Input: part model. Units: mm. Frame: model coordinates. Give positions to 0.01 mm unless a question says otherwise; leave off trailing zeros. Loops run counter-clockwise (first coordinate to the right, second up) from the corner with the lowest first, then second, coordinate; pieces in that order, holes last. Notation, with made-up numbers: (39, 73.25) - (85, 73.25) arc R21 cw to (85, 98.25) - close; hole circle Ø10 at (0.5, -25.5). An arc over 180 degrees is marked (long way). One line per item, written item: value.
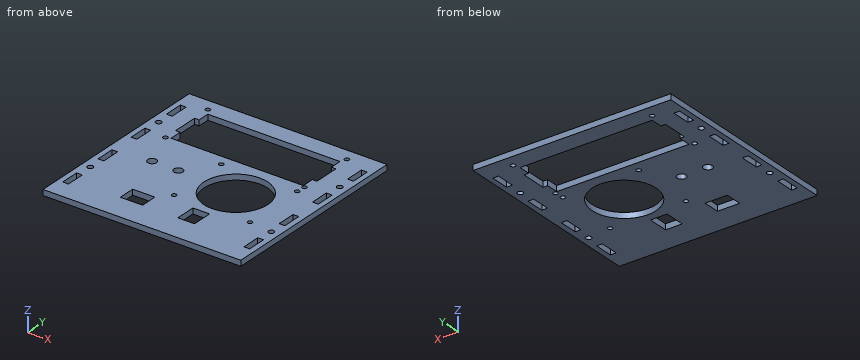
Autodesk Inventor part; units mm, degrees
ref_plane "YZ Plane" through (0, 0, 0) normal (1, 0, 0) x (0, 1, 0)
ref_plane "XZ Plane" through (0, 0, 0) normal (0, 1, 0) x (-1, 0, 0)
ref_plane "XY Plane" through (0, 0, 0) normal (0, 0, 1) x (1, 0, 0)
sketch "Sketch1" plane through (0, 0, 0) normal (0, 0, 1) x (1, 0, 0)
  line L0 (-51.5546, 67.657) -> (55.1254, 67.657)
  line L1 (55.1254, 67.657) -> (55.1254, -39.023)
  line L2 (55.1254, -39.023) -> (-51.5546, -39.023)
  line L3 (-51.5546, -39.023) -> (-51.5546, 67.657)
  dimension "d0" = 106.68
  dimension "d2" = 106.68
extrude "Extrusion1" add sketch "Sketch1" against normal blind 3
sketch "LCD Cut Out" plane through (0, 0, 0) normal (0, 0, 1) x (1, 0, 0)
  circle A0 centre (-36.5621, 61.0277) radius 1.25
  circle A1 centre (-36.5621, 30.0277) radius 1.25
  circle A2 centre (38.4379, 61.0277) radius 1.25
  circle A3 centre (38.4379, 30.0277) radius 1.25
  line L0 (-34.1482, 57.6923) -> (37.1518, 57.6923)
  line L1 (37.1518, 57.6923) -> (37.1518, 30.8923)
  line L2 (37.1518, 30.8923) -> (-34.1482, 30.8923)
  line L3 (-34.1482, 30.8923) -> (-34.1482, 57.6923)
  line L4 (37.1196, 51.3389) -> (39.6196, 51.3389)
  line L5 (39.6196, 51.3389) -> (39.6196, 37.5389)
  line L6 (39.6196, 37.5389) -> (37.1196, 37.5389)
  line L7 (37.1196, 37.5389) -> (37.1196, 51.3389)
  line L8 (-36.6336, 51.3389) -> (-34.1336, 51.3389)
  line L9 (-34.1336, 51.3389) -> (-34.1336, 37.5389)
  line L10 (-34.1336, 37.5389) -> (-36.6336, 37.5389)
  line L11 (-36.6336, 37.5389) -> (-36.6336, 51.3389)
  point P0 (0, 0)
  dimension "d96" = 76.2532
sketch "Sketch9" plane through (0, 0, 0) normal (0, 0, 1) x (1, 0, 0)
  circle A0 centre (-14.4313, 9.525) radius 2.4
  circle A1 centre (-28.575, 9.525) radius 2.4
  circle A2 centre (17.7335, 7.9375) radius 17.2
  circle A3 centre (-2.8375, 25.1375) radius 1.25
  circle A4 centre (38.1, 25.1375) radius 1.25
  circle A5 centre (38.1, -9.2625) radius 1.25
  circle A6 centre (-2.8375, -9.2625) radius 1.25
  line L0 (-20.4313, -15.698) -> (-8.4313, -15.698)
  line L1 (-8.4313, -15.698) -> (-8.4313, -24.698)
  line L2 (-8.4313, -24.698) -> (-20.4313, -24.698)
  line L3 (-20.4313, -24.698) -> (-20.4313, -15.698)
  line L4 (10.5687, -13.698) -> (19.5687, -13.698)
  line L5 (19.5687, -13.698) -> (19.5687, -24.698)
  line L6 (19.5687, -24.698) -> (10.5687, -24.698)
  line L7 (10.5687, -24.698) -> (10.5687, -13.698)
  line L8 (-51.5546, 67.657) -> (55.1254, 67.657)
  line L9 (55.1254, -39.023) -> (-51.5546, -39.023)
  line L10 (55.1254, 67.657) -> (55.1254, -39.023)
  circle A7 centre (-47.0546, 39.257) radius 1.525
  circle A8 centre (-47.0546, -10.623) radius 1.525
  circle A9 centre (50.6254, 39.257) radius 1.525
  circle A10 centre (50.6254, -10.623) radius 1.525
  line L11 (-48.6128, 57.182) -> (-45.5128, 57.182)
  line L12 (-45.5128, 57.182) -> (-45.5128, 47.082)
  line L13 (-45.5128, 47.082) -> (-48.6128, 47.082)
  line L14 (-48.6128, 47.082) -> (-48.6128, 57.182)
  line L15 (-45.5506, 31.432) -> (-48.6506, 31.432)
  line L16 (-48.6506, 31.432) -> (-48.6506, 21.332)
  line L17 (-48.6506, 21.332) -> (-45.5506, 21.332)
  line L18 (-45.5506, 21.332) -> (-45.5506, 31.432)
  line L19 (-45.5506, -2.798) -> (-48.6506, -2.798)
  line L20 (-48.6506, -2.798) -> (-48.6506, 7.302)
  line L21 (-48.6506, 7.302) -> (-45.5506, 7.302)
  line L22 (-45.5506, 7.302) -> (-45.5506, -2.798)
  line L23 (-45.5506, -18.448) -> (-48.6506, -18.448)
  line L24 (-48.6506, -18.448) -> (-48.6506, -28.548)
  line L25 (-48.6506, -28.548) -> (-45.5506, -28.548)
  line L26 (-45.5506, -28.548) -> (-45.5506, -18.448)
  line L27 (52.0999, 7.3659) -> (48.9999, 7.3659)
  line L28 (48.9999, 7.3659) -> (48.9999, -2.7341)
  line L29 (48.9999, -2.7341) -> (52.0999, -2.7341)
  line L30 (52.0999, -2.7341) -> (52.0999, 7.3659)
  line L31 (52.1638, -18.4611) -> (49.0638, -18.4611)
  line L32 (49.0638, -18.4611) -> (49.0638, -28.5611)
  line L33 (49.0638, -28.5611) -> (52.1638, -28.5611)
  line L34 (52.1638, -28.5611) -> (52.1638, -18.4611)
  line L35 (52.2687, 46.9823) -> (49.1687, 46.9823)
  line L36 (49.1687, 46.9823) -> (49.1687, 57.0823)
  line L37 (49.1687, 57.0823) -> (52.2687, 57.0823)
  line L38 (52.2687, 57.0823) -> (52.2687, 46.9823)
  line L39 (52.2687, 31.4608) -> (49.1687, 31.4608)
  line L40 (49.1687, 31.4608) -> (49.1687, 21.3608)
  line L41 (49.1687, 21.3608) -> (52.2687, 21.3608)
  line L42 (52.2687, 21.3608) -> (52.2687, 31.4608)
  point P0 (0, 0)
  dimension "d56" = 4.8
  dimension "d57" = 4.8
  dimension "d60" = 34.4
  dimension "d62" = 2.5
  dimension "d63" = 2.5
  dimension "d64" = 2.5
  dimension "d65" = 2.5
  dimension "d66" = 12
  dimension "d67" = 9
  dimension "d69" = 9
  dimension "d70" = 11
  dimension "d72" = 40
  dimension "d88" = 3.05
  dimension "d89" = 28.4
  dimension "d91" = 3.05
  dimension "d92" = 28.4
  dimension "d93" = 3.05
  dimension "d95" = 3.05
  dimension "d98" = 3.1
  dimension "d99" = 10.1
  dimension "d100" = 3.1
  dimension "d101" = 10.1
  dimension "d102" = 6.3
  dimension "d103" = 6.3
  dimension "d104" = 3.1
  dimension "d105" = 10.1
  dimension "d106" = 3.1
  dimension "d107" = 10.1
  dimension "d108" = 6.3
  dimension "d109" = 6.3
  dimension "d110" = 3.1
  dimension "d111" = 10.1
  dimension "d112" = 3.1
  dimension "d113" = 10.1
  dimension "d117" = 4.5
  dimension "d120" = 3.1
  dimension "d121" = 10.1
  dimension "d122" = 3.1
  dimension "d123" = 10.1
  dimension "d126" = 14.325
  dimension "d127" = 14.325
extrude "Extrusion4" cut sketch "Sketch9" against normal blind 28.4
extrude "Extrusion5" cut sketch "LCD Cut Out" against normal blind 3
equation "\"d75\" = d89"
properties part number "open reflow box"
Item 1: Material intervals for L1, parallel to X at y = -25.5, z = -1.15; L2, parallel to Y at x = -11, z = -0.1; L3, parallel to Y at x = 21, z = -0.5, sorted ascending.
Verdict:
L1: x = -51.55 to -48.65, -45.55 to 49.06, 52.16 to 55.13
L2: y = -39.02 to -24.7, -15.7 to 30.89, 57.69 to 67.66
L3: y = -39.02 to -8.95, 24.82 to 30.89, 57.69 to 67.66
Item 2: Pin query (flat end, axial travel): P1, Ø2, axis at x = 38.1, y = 25.14, coming from the +Z side. Return the tip coordinate at first contact, or that it passes through.
Verdict:
P1: passes through
Item 3: Section D-D, the plane x = 2. Output: boundary loops of the cut face in (y, z).
Verdict:
outline: (-39.02, -3) - (0.99, -3) - (0.99, 0) - (-39.02, 0) - close; (14.89, -3) - (30.89, -3) - (30.89, 0) - (14.89, 0) - close; (57.69, -3) - (67.66, -3) - (67.66, 0) - (57.69, 0) - close
Item 4: Section B-B, the plane x = 22. Output: boundary loops of the cut face in (y, z), and give its area (3 significant figures).
Verdict:
outline: (-39.02, -3) - (-8.72, -3) - (-8.72, 0) - (-39.02, 0) - close; (24.6, -3) - (30.89, -3) - (30.89, 0) - (24.6, 0) - close; (57.69, -3) - (67.66, -3) - (67.66, 0) - (57.69, 0) - close
area: 140 mm^2
Item 5: Section C-C, the plane z = -0.9. Count the separate pieces of the cut face and the enclosed holes in it, and give its area (3 significant figures).
Verdict:
separate pieces: 1
enclosed holes: 26
area: 7,910 mm^2
Item 6: Section A-A, the plane y = 53.5. Output: boundary loops of the cut face in (x, z), and give its area (3 significant figures).
Verdict:
outline: (-51.55, -3) - (-48.61, -3) - (-48.61, 0) - (-51.55, 0) - close; (-45.51, -3) - (-34.15, -3) - (-34.15, 0) - (-45.51, 0) - close; (37.15, -3) - (49.17, -3) - (49.17, 0) - (37.15, 0) - close; (52.27, -3) - (55.13, -3) - (55.13, 0) - (52.27, 0) - close
area: 87.5 mm^2
